Autodesk Inventor part; units mm, degrees
ref_plane "YZ Plane" through (0, 0, 0) normal (1, 0, 0) x (0, 1, 0)
ref_plane "XZ Plane" through (0, 0, 0) normal (0, 1, 0) x (-1, 0, 0)
ref_plane "XY Plane" through (0, 0, 0) normal (0, 0, 1) x (1, 0, 0)
sketch "Sketch1" plane through (0, 0, 0) normal (1, 0, 0) x (0, 1, 0)
  line L0 (0, 0) -> (25, 0)
  line L1 (25, 0) -> (25, -25)
  line L2 (25, -25) -> (0, -25)
  line L3 (0, -25) -> (0, 0)
  line L4 (3, -3) -> (22, -3)
  line L5 (22, -3) -> (22, -22)
  line L6 (22, -22) -> (3, -22)
  line L7 (3, -22) -> (3, -3)
  dimension "d0" = 25
  dimension "d1" = 25
  dimension "d2" = 3
extrude "Extrusion1" add sketch "Sketch1" along normal blind 590
sketch "Sketch2" plane through (0, 0, 0) normal (0, 0, 1) x (1, 0, 0)
  line L0 (0, 25) -> (590, 25)
  line L1 (0, 0) -> (590, 0)
  point P0 (20, 12.5)
  point P1 (570, 12.5)
  point P2 (295, 25)
  dimension "d5" = 550
  dimension "d6" = 275
  dimension "d7" = 12.5
  dimension "d15" = 12.5
hole "Hole1" at (20, 12.5, 0) at (570, 12.5, 0) direction (0, 0, -1) diameter 12 end through all
properties part number "P001" material "Aluminum 6061"
Part model, mm, in its own coordinate system. A direction names the side the tool comes from. Round coordinates to 2 decimals unless told otherwise and drop trailing zeros. Order: outer loops, then holes, each group sorted by start corner. A loop starts at its lowest first (then second) coordinate and runs counter-clockwise, first axis right, second up. Notation, with made-up numbers: M 49.25,-21.75 L 96.25,-21.75 A30 ccw 96.25,16.25 Z; hole C 63,28.5 d10. An arc over 180 degrees is marked long. Answer in a Markdown table with one row per item. Add a question column.
Q1. 3-axis set-ups, long thin cutter, end or side, ignore diameter. For faces 1 (the face through (291, 3, -13)), 2 (the face through (0, 23, -12)): which of +Z, -Z, +X, -X, +Y, -Y reach the whole face in a straight line?
Q2. Mould opens along Z. For faces 3 (the face through (291, 22, -12)), 4 (the face through (291, 12, 0)), 5 (the face through (291, 0, -13)) say: +Z half, -Z half, draft (parallel to the pull), parting line (faces both ways), or undercut.
Q3. Cut at C-C on y = 12.5. Give the cut face in (x, z).
Q4. Wall check: L1, parallel to X at y = 12.5, z = -0.65; L2, parallel to Y at x = 570, z = -1.6; L3, parallel to Z at x = 272, y = 13.75. Give the ranges that are in metal, low to high. Write a range as from..to.
Q5. Cut at B-B on z = -16.75. Give the cut face in (x, y), and give its area (3 significant figures).
Q6. Cut at A-A on x = 570. Give the cut face in (y, z).
Q7. Cut at D-D on x = 213. Give the cut face in (y, z).
Established:
| question | item | result |
|---|---|---|
| 1 | face 1 | +X, -X |
| 1 | face 2 | +Z, -Z, -X, +Y, -Y |
| 2 | face 3 | undercut |
| 2 | face 4 | +Z half |
| 2 | face 5 | draft |
| 3 | outline | M 0,-25 L 14,-25 L 14,-22 L 0,-22 Z; M 0,-3 L 14,-3 L 14,0 L 0,0 Z; M 26,-25 L 564,-25 L 564,-22 L 26,-22 Z; M 26,-3 L 564,-3 L 564,0 L 26,0 Z; M 576,-25 L 590,-25 L 590,-22 L 576,-22 Z; M 576,-3 L 590,-3 L 590,0 L 576,0 Z |
| 4 | L1 | x = 0..14, 26..564, 576..590 |
| 4 | L2 | y = 0..6.5, 18.5..25 |
| 4 | L3 | z = -25..-22, -3..0 |
| 5 | outline | M 0,0 L 590,0 L 590,3 L 0,3 Z; M 0,22 L 590,22 L 590,25 L 0,25 Z |
| 5 | area | 3,540 mm2 |
| 6 | outline | M 0,-25 L 6.5,-25 L 6.5,-22 L 3,-22 L 3,-3 L 6.5,-3 L 6.5,0 L 0,0 Z; M 18.5,-25 L 25,-25 L 25,0 L 18.5,0 L 18.5,-3 L 22,-3 L 22,-22 L 18.5,-22 Z |
| 7 | outline | M 0,-25 L 25,-25 L 25,0 L 0,0 Z; hole M 3,-22 L 22,-22 L 22,-3 L 3,-3 Z |
